Model file for the job. Use its own axes, mm. Face numbers are marked on the shaded views. Give positions to 0.01 mm unless a question says otherwise; leave off trailing zeros. Order: outer loops, then holes, each group sorted by start corner. A loop starts at its lowest first (then second) coordinate and runs counter-clockwise, first axis right, second up. Notation, with made-up numbers: M -7,31.5 L 48,31.5 A17 ccw 48,44.5 Z; hole C -26.75,37.5 d11. An arc over 180 degrees is marked long. Return JSON: item names as keys, results as strings. Group by question number.
1. Slice it at C-C on z = 46. List the corners of the cut face in (x, y).
2. Slice it at B-B on x = 114. List the corners of the cut face in (y, z), then the cut area to 3 significant figures.
3. Two-plate mould, pull along X, no slides. Class the marked faces 1 and 2: released by +X, released by -X, zero draft, split by the parting line, or undercut.
4. Pin check, flat tips, straight feed: pin 1 (2 mm diameter, centred on x = 105, y = 30, fed in from +Z); pin 2 (10 mm diameter, centred on x = 107.5, z = 24, fed in from +Y); pin 3 (12 mm diameter, centred on x = -38.5, y = 4, fed in from +Z). Stop position of each tip, or through.
5. Wall check: probe 1 along X at (y, z) = (26, 16); probe 2 along X at (y, z) = (1.5, -8); probe 3 along Y at (x, z) = (37.5, 36). Give the ranges that are in metal, low to high. Write a range as [from, to].
6. Slice it at A-A on x = 13. List the corners of the cut face in (y, z), then the cut area to 3 significant figures.
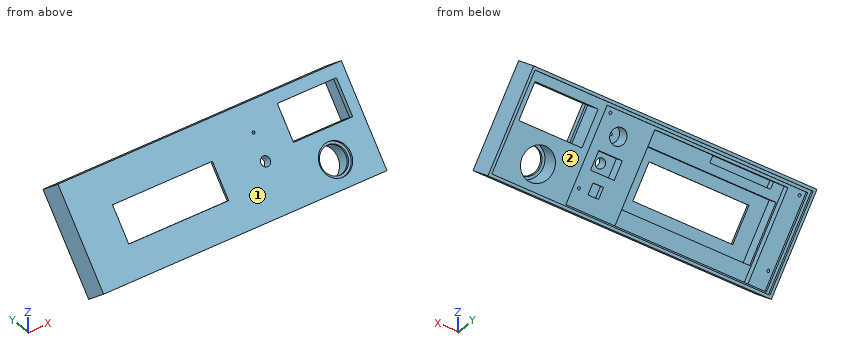
from build123d import *

# Parameters (mm, degrees)
F3_W      = 215.6
F3_H      = 72.8
F4_DEPTH  = 20
F5_W      = 76
F5_H      = 26
F5_R      = 3.5
F6_DEPTH  = 55.8480022096
F7_R      = 1
F8_DEPTH  = 18
F9_W      = 99.2
F9_H      = 41.8
F10_DEPTH = 18
F11_R     = 6
F11_R_2   = 1
F12_DEPTH = 14
F13_DEPTH = 55.8480022096
F14_W     = 18
F14_H     = 13
F15_DEPTH = 12
F16_W     = 8
F16_H     = 8
F17_DEPTH = 8
F18_W     = 101.2
F18_H     = 63.8
F19_DEPTH = 9
F20_W     = 46.2
F20_H     = 5
F22_DEPTH = 5
F23_W     = 152.6
F23_H     = 65.8
F24_DEPTH = 4
F25_W     = 45
F25_H     = 25.8
F26_DEPTH = 55.8480022096
F27_W     = 48
F27_H     = 25.8
F28_DEPTH = 16
F29_R     = 10
F30_DEPTH = 55.8480022096
F29_R_2   = 11.75
F31_DEPTH = 2
F32_R     = 12
F33_DEPTH = 16
F34_W     = 211.6
F34_H     = 68.8
F35_DEPTH = 2


with BuildPart() as f4:
    # F3 (on face) → F4 (new body)
    with BuildSketch(Plane(origin=(0, -4.9240387651, 4.1317591117), x_dir=(-1, 0, 0), z_dir=(0, 0.7660444431, -0.6427876097))):
        with Locations((-33.6366042773, 23.835632431)):
            Rectangle(F3_W, F3_H)
    extrude(amount=F4_DEPTH)

    # F5 (on face) → F6 (cut, through all)
    with BuildSketch(Plane(origin=(0, -4.9240387651, 4.1317591117), x_dir=(1, 0, 0), z_dir=(0, -0.7660444431, 0.6427876097))):
        with Locations((-6.5633957227, 22.335632431)):
            Rectangle(F5_W, F5_H)
        with Locations((65.6750798225, 22.335632431)):
            Circle(F5_R)
    extrude(amount=-F6_DEPTH, mode=Mode.SUBTRACT)

    # F7 (on face) → F8 (cut, through all)
    with BuildSketch(Plane(origin=(0, 10.3968500973, -8.7239930821), x_dir=(-1, 0, 0), z_dir=(0, 0.7660444431, -0.6427876097))):
        with Locations((-77.2366042773, 52.835632431)):
            Circle(F7_R)
        with Locations((-77.2366042773, 2.835632431)):
            Circle(F7_R)
        with Locations((66.7633957227, 2.835632431)):
            Circle(F7_R)
        with Locations((66.7633957227, 52.835632431)):
            Circle(F7_R)
    extrude(amount=-F8_DEPTH, mode=Mode.SUBTRACT)

    # F9 (on face) → F10 (cut, through all)
    with BuildSketch(Plane(origin=(0, 10.3968500973, -8.7239930821), x_dir=(-1, 0, 0), z_dir=(0, 0.7660444431, -0.6427876097))):
        with Locations((6.5633957227, 22.335632431)):
            Rectangle(F9_W, F9_H)
    extrude(amount=-F10_DEPTH, mode=Mode.SUBTRACT)

    # F11 (on face) → F12 (cut, through all)
    with BuildSketch(Plane(origin=(0, 10.3968500973, -8.7239930821), x_dir=(-1, 0, 0), z_dir=(0, 0.7660444431, -0.6427876097))):
        with Locations((-65.6750798225, 41.335632431)):
            Circle(F11_R)
        with Locations((-65.6750798225, 41.335632431)):
            Circle(F11_R_2, mode=Mode.SUBTRACT)
        with Locations((-65.6750798225, 41.335632431)):
            Circle(F11_R_2)
    extrude(amount=-F12_DEPTH, mode=Mode.SUBTRACT)

    # F11 (on face) → F13 (cut, through all)
    with BuildSketch(Plane(origin=(0, 10.3968500973, -8.7239930821), x_dir=(-1, 0, 0), z_dir=(0, 0.7660444431, -0.6427876097))):
        with Locations((-65.6750798225, 41.335632431)):
            Circle(F11_R_2)
    extrude(amount=-F13_DEPTH, mode=Mode.SUBTRACT)

    # F14 (on face) → F15 (cut, through all)
    with BuildSketch(Plane(origin=(0, 10.3968500973, -8.7239930821), x_dir=(-1, 0, 0), z_dir=(0, 0.7660444431, -0.6427876097))):
        with Locations((-65.6750798225, 22.335632431)):
            Rectangle(F14_W, F14_H)
    extrude(amount=-F15_DEPTH, mode=Mode.SUBTRACT)

    # F16 (on face) → F17 (cut, through all)
    with BuildSketch(Plane(origin=(0, 10.3968500973, -8.7239930821), x_dir=(-1, 0, 0), z_dir=(0, 0.7660444431, -0.6427876097))):
        with Locations((-65.6750798225, 5.335632431)):
            Rectangle(F16_W, F16_H)
    extrude(amount=-F17_DEPTH, mode=Mode.SUBTRACT)

    # F18 (on face) → F19 (cut, through all)
    with BuildSketch(Plane(origin=(0, 10.3968500973, -8.7239930821), x_dir=(-1, 0, 0), z_dir=(0, 0.7660444431, -0.6427876097))):
        with Locations((6.5633957227, 22.335632431)):
            Rectangle(F18_W, F18_H)
    extrude(amount=-F19_DEPTH, mode=Mode.SUBTRACT)

    # F20 (on face) → F22 (cut)
    with BuildSketch(Plane(origin=(0, 3.5024501092, -2.9389045949), x_dir=(-1, 0, 0), z_dir=(0, 0.7660444431, -0.6427876097))):
        with Locations((26.0633957227, 51.735632431)):
            Rectangle(F20_W, F20_H)
    extrude(amount=-F22_DEPTH, mode=Mode.SUBTRACT)

    # F23 (on face) → F24 (cut, through all)
    with BuildSketch(Plane(origin=(0, 10.3968500973, -8.7239930821), x_dir=(-1, 0, 0), z_dir=(0, 0.7660444431, -0.6427876097))):
        with Locations((-6.1366042773, 23.335632431)):
            Rectangle(F23_W, F23_H)
    extrude(amount=-F24_DEPTH, mode=Mode.SUBTRACT)

    # F25 (on face) → F26 (cut, through all)
    with BuildSketch(Plane(origin=(0, -4.9240387651, 4.1317591117), x_dir=(-1, 0, 0), z_dir=(0, 0.7660444431, -0.6427876097))):
        with Locations((-111.2485080957, 38.9576355718)):
            Rectangle(F25_W, F25_H)
    extrude(amount=F26_DEPTH, mode=Mode.SUBTRACT)

    # F27 (on face) → F28 (cut, through all)
    with BuildSketch(Plane(origin=(0, 10.3968500973, -8.7239930821), x_dir=(-1, 0, 0), z_dir=(0, 0.7660444431, -0.6427876097))):
        with Locations((-111.2485080957, 38.9576355718)):
            Rectangle(F27_W, F27_H)
    extrude(amount=-F28_DEPTH, mode=Mode.SUBTRACT)

    # F29 (on face) → F30 (cut, through all)
    with BuildSketch(Plane(origin=(0, -4.9240387651, 4.1317591117), x_dir=(-1, 0, 0), z_dir=(0, 0.7660444431, -0.6427876097))):
        with Locations((-111.2485080957, 6.2527651899)):
            Circle(F29_R)
    extrude(amount=F30_DEPTH, mode=Mode.SUBTRACT)

    # F29 (on face) → F31 (cut)
    with BuildSketch(Plane(origin=(0, -4.9240387651, 4.1317591117), x_dir=(-1, 0, 0), z_dir=(0, 0.7660444431, -0.6427876097))):
        with Locations((-111.2485080957, 6.2527651899)):
            Circle(F29_R_2)
        with Locations((-111.2485080957, 6.2527651899)):
            Circle(F29_R, mode=Mode.SUBTRACT)
    extrude(amount=F31_DEPTH, mode=Mode.SUBTRACT)

    # F32 (on face) → F33 (cut, through all)
    with BuildSketch(Plane(origin=(0, 10.3968500973, -8.7239930821), x_dir=(-1, 0, 0), z_dir=(0, 0.7660444431, -0.6427876097))):
        with Locations((-111.2485080957, 6.2527651899)):
            Circle(F32_R)
    extrude(amount=-F33_DEPTH, mode=Mode.SUBTRACT)

    # F34 (on face) → F35 (cut)
    with BuildSketch(Plane(origin=(0, 10.3968500973, -8.7239930821), x_dir=(-1, 0, 0), z_dir=(0, 0.7660444431, -0.6427876097))):
        with Locations((-33.6366042773, 23.835632431)):
            Rectangle(F34_W, F34_H)
    extrude(amount=-F35_DEPTH, mode=Mode.SUBTRACT)


solid = f4.part
Result:
{
 "1": {"outline": "M -74.16,30.21 L 141.44,30.21 L 141.44,38.89 L -74.16,38.89 Z"},
 "2": {"outline": "M -13,-5.49 L 2.32,-18.35 L 3.61,-16.82 L 2.07,-15.53 L 5.38,-11.6 L -5.35,-2.6 L -4.02,-1.01 L -5.55,0.27 L -6.72,-1.11 L -8.25,0.17 Z; M 6.44,17.67 L 7.97,16.39 L 6.81,15 L 8.34,13.72 L 9.67,15.3 L 20.39,6.3 L 25.61,12.52 L 11.83,24.09 Z; M 28.41,43.86 L 42.2,32.29 L 46.3,37.17 L 47.83,35.89 L 49.12,37.42 L 33.79,50.27 Z", "area": "443 mm2"},
 "3": {"face 1": "zero draft", "face 2": "undercut"},
 "4": {"pin 1": "stops at z = 46.94", "pin 2": "stops at y = 17.9", "pin 3": "stops at z = 11.28"},
 "5": {"probe 1": "x = [-74.16, -70.16], [82.44, 87.25], [135.25, 141.44]", "probe 2": "x = [-74.16, -57.16], [44.04, 107.55], [114.94, 141.44]", "probe 3": "y = [21.82, 36.18], [41.47, 42.7], [44.58, 45.31], [47.7, 47.92]"},
 "6": {"outline": "M -13,-5.49 L 2.32,-18.35 L 3.61,-16.82 L 2.07,-15.53 L 2.72,-14.77 L -2.65,-10.27 L 4.43,-1.84 L -2.47,3.95 L 2.61,10 L 1.08,11.28 Z; M 17.79,31.2 L 19.32,29.91 L 24.4,35.97 L 31.29,30.18 L 38.36,38.61 L 42.19,35.39 L 43.48,36.93 L 45.01,35.64 L 46.3,37.17 L 47.83,35.89 L 49.12,37.42 L 33.79,50.27 Z", "area": "440 mm2"}
}
